Job drawing, mm, ordinate dimensions from the low corner. One solid piece. A direction names the side the tool comes from. Give positions to 0.01 mm unless a question says otherwise; leave off trailing zeros. Loops run counter-clockwise (first coordinate to the right, second up) from the corner with the lowest first, then second, coordinate; pieces in that order, holes last.
Item 1: Saw through at A-A on z = 10.5. Give the number of separate pieces and of enclosed holes in the cut face, plus the area to 3 significant figures.
Item 2: Probe probe 1 along X at (y, z) = (1.5, 12.75); probe 2 along Y at (x, z) = (51, 1.75); probe 3 along Z at (x, y) = (9, 9.75). List the from-to ranges inside material, lowest first.
Item 3: Which spindle directions (+Z, -Z, +X, -X, +Y, -Y) get a long thin tool onto all of the face, cutting with end or side? Do the marked faces 5, 6 and 7. Say none if no direction does.
Item 4: Saw through at C-C on x = 51.5. Give the cut face in (y, z).
Item 5: Mould opens along X. For the marked faces 1, 2, 3 and 4 say: released by +X, released by -X, zero draft, split by the parting line, or undercut.
Item 6: Drop flat-ended pins along their axis: P1, Ø2, axis at x = 15.5, z = 15, coming from the +Y side; P2, Ø8, axis at x = 58, z = 10.5, coming from the +Y side; P3, Ø1.5, axis at y = 22, z = 7.5, coming from the -X side; P4, Ø7.5, axis at x = 9.525, z = 9.525, coming from the +Y side. Give the stop position or say it passes through.
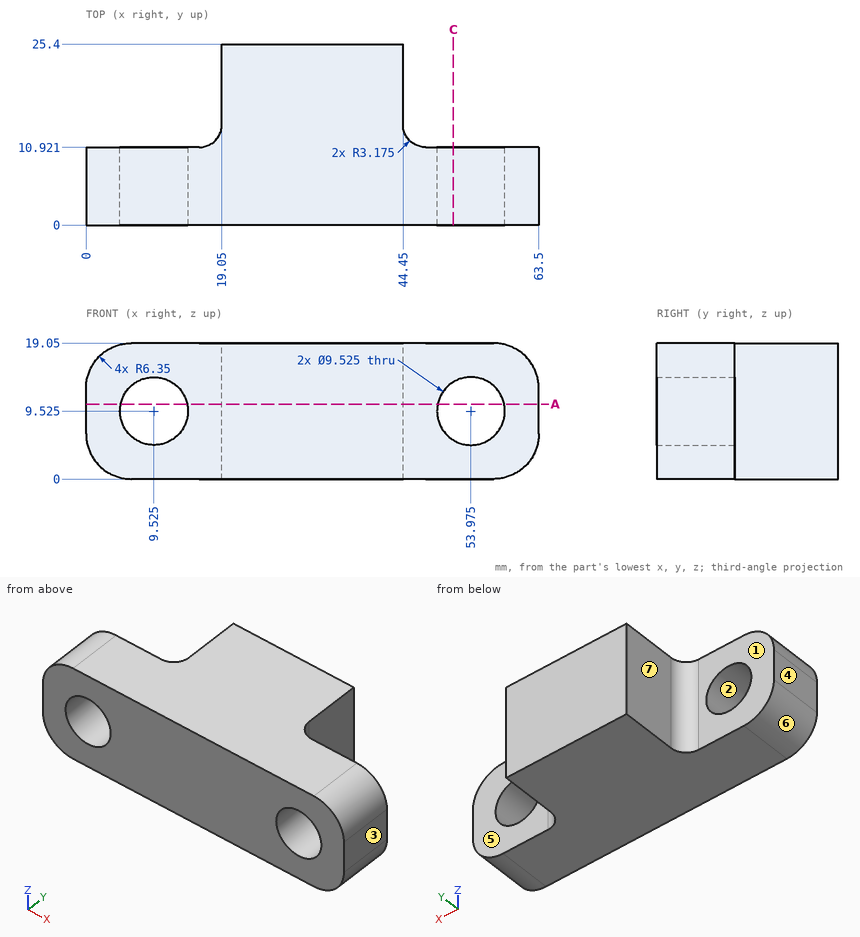
Results below:
1. separate pieces: 3
1. enclosed holes: 0
1. area: 862 mm2
2. probe 1: x = 0 to 6.02, 13.03 to 50.47, 57.48 to 63.5
2. probe 2: y = 0 to 10.92
2. probe 3: z = 0 to 4.79, 14.26 to 19.05
3. face 5: +Z, -Z, +X, +Y
3. face 6: -Z, -X, +Y, -Y
3. face 7: +Z, -Z, -X, +Y
4. outline: (0, 0) - (10.92, 0) - (10.92, 5.46) - (0, 5.46) - close; (0, 13.59) - (10.92, 13.59) - (10.92, 19.05) - (0, 19.05) - close
5. face 1: zero draft
5. face 2: undercut
5. face 3: released by +X
5. face 4: released by -X
6. P1: stops at y = 10.98
6. P2: stops at y = 10.92
6. P3: stops at x = 19.05
6. P4: passes through
